Geometry check sheet. Reference: the model listing, model coordinates, mm. Coordinates: 2 decimals unless noted, no trailing zeros. Loops run counter-clockwise (first coordinate to the right, second up) from the corner with the lowest first, then second, coordinate; pieces in that order, holes last.
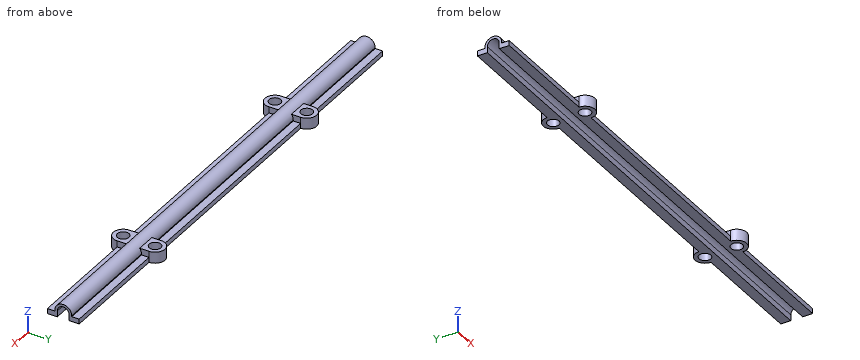
Autodesk Fusion 360 part; units mm, degrees
sketch "Sketch1" plane through (0, 0, 0) normal (1, 0, 0) x (0, 1, 0) in component "CAN_Cable_Cover"
  circle A0 centre (0, 2.4) radius 2.4
  line L0 (-2.4, 2.4) -> (-2.4, 0)
  line L1 (0, 2.5) -> (0, 20)
  line L2 (2.4, 2.4) -> (2.4, 0)
  circle A1 centre (0, 2.4) radius 3.4
  line L3 (-3.4, 2.4) -> (-3.4, 0)
  line L4 (-3.4, 0) -> (-2.4, 0)
  line L5 (3.4, 2.4) -> (3.4, 0)
  line L6 (3.4, 0) -> (2.4, 0)
  line L7 (-3.4, 0) -> (-6.4, 0)
  line L8 (-6.4, 0) -> (-6.4, 2)
  line L9 (-6.4, 2) -> (-3.4, 2)
  line L10 (-3.4, 2) -> (-3.4, 0)
  line L11 (6.4, 2) -> (3.4, 2)
  line L12 (6.4, 0) -> (6.4, 2)
  line L13 (3.4, 0) -> (6.4, 0)
  line L14 (3.4, 2) -> (3.4, 0)
  dimension "d1" = 4.8
  dimension "d2" = 1
  dimension "d5" = 3
  dimension "d6" = 2
extrude "Extrude1" add sketch "Sketch1" along normal mid plane 200 contours A0 L0 L1 A1 L4 | A0 L1 L2 A1 L6 | A1 L3 L4 L10 | A1 L5 L6 L14 | L3 L7 L8 L9 L10 | L5 L11 L12 L13 L14 in component "CAN_Cable_Cover"
sketch "Sketch2" plane through (0, 0, 0) normal (0, 0, -1) x (1, 0, 0) in component "CAN_Cable_Cover"
  line L0 (-100, 2.4) -> (100, 2.4)
  line L1 (100, 2.4) -> (100, 6.4)
  line L2 (100, 6.4) -> (-100, 6.4)
  line L3 (-100, 6.4) -> (-100, 2.4)
  circle A0 centre (-50, 6.4) radius 4
  line L4 (0, -1.75) -> (0, -22.5)
  circle A1 centre (-50, 6.4) radius 2.35
  line L5 (-46, 6.4) -> (-46, 2.4)
  line L6 (-46, 2.4) -> (-50, 2.4)
  line L7 (-54, 6.4) -> (-54, 2.4)
  line L8 (-54, 2.4) -> (-50, 2.4)
  line L9 (1.75, 0) -> (22.5, 0)
  circle A2 centre (-50, -6.4) radius 4
  circle A3 centre (-50, -6.4) radius 2.35
  line L10 (-54, -6.4) -> (-54, -2.4)
  line L11 (-54, -2.4) -> (-50, -2.4)
  line L12 (-46, -2.4) -> (-50, -2.4)
  line L13 (-46, -6.4) -> (-46, -2.4)
  line L14 (46, -2.4) -> (50, -2.4)
  line L15 (54, 6.4) -> (54, 2.4)
  line L16 (54, 2.4) -> (50, 2.4)
  line L17 (46, 6.4) -> (46, 2.4)
  circle A4 centre (50, 6.4) radius 4
  circle A5 centre (50, -6.4) radius 4
  line L18 (54, -6.4) -> (54, -2.4)
  circle A6 centre (50, -6.4) radius 2.35
  line L19 (46, -6.4) -> (46, -2.4)
  circle A7 centre (50, 6.4) radius 2.35
  line L20 (54, -2.4) -> (50, -2.4)
  line L21 (46, 2.4) -> (50, 2.4)
  dimension "d7" = 8
  dimension "d8" = 50
  dimension "d9" = 4.7
extrude "Extrude2" add sketch "Sketch2" against normal blind 4.5 contours L0 A0 L7 L8 | L0 A0 L5 L6 | L2 A0 A1 | L2 A0 A1 | L0 L17 A4 L21 | L2 A4 A7 | L2 A4 A7 | L0 L15 L16 A4 | A2 | A2 L12 L13 | A2 L10 L11 | L14 A5 L19 | A5 L18 L20 | A5 in component "CAN_Cable_Cover"
extrude "Extrude3" cut sketch "Sketch2" against normal blind 16 contours L2 A1 | L2 A7 | A3 | A6 picked at (-50.2862, 5.6708) picked at (49.2594, 5.8292) in component "CAN_Cable_Cover"
component "CAN_Cable_Cover" placed x (1, 0, 0) y (0, 1, 0) z (0, 0, 1) at (0, 0, 0)
equation "d1 = cable_dia"
equation "d2 = tube_thick"
equation "d3 = length"
equation "d4 = 0deg 0'"
equation "d11 = 0deg 0'"
equation "d13 = 0deg 0'"
equation "length = 200 mm"
equation "cable_dia = 4.8 mm"
equation "tube_thick = 1 mm"
1) Depth check by flat-ended pin: pin 1 (6 mm diameter, centred on x = -50, y = -6.4, fed in from +Z); pin 2 (1.2 mm diameter, centred on x = 11, z = 1, fed in from -Y); pin 3 (1.9 mm diameter, centred on x = 41, z = 1.5, fed in from +Y). Enter the tip coordinate at first touch or a pass-through.
Data:
pin 1: stops at z = 4.5
pin 2: stops at y = -6.4
pin 3: stops at y = 6.4
2) Material ranges on probe 1 along Y at (x, z) = (50, 1.55); probe 2 along X at (y, z) = (6.4, 2.8); probe 3 along X at (y, z) = (3, 4.4), recorded low to high.
Data:
probe 1: y = -10.4 to -8.75, -4.05 to -2.4, 2.4 to 4.05, 8.75 to 10.4
probe 2: x = -54 to -52.35, -47.65 to -46, 46 to 47.65, 52.35 to 54
probe 3: x = -54 to -46, 46 to 54
3) Section check B-B on y = 0. Record the cut outline in (x, z).
Data:
outline: (-100, 4.8) - (100, 4.8) - (100, 5.8) - (-100, 5.8) - close
4) Section check A-A on x = 50. Record the cut outline in (y, z), and give its area (3 significant figures).
Data:
outline: (-10.4, 0) - (-8.75, 0) - (-8.75, 4.5) - (-10.4, 4.5) - close; (-4.05, 0) - (-2.4, 0) - (-2.4, 2.4) arc R2.4 cw to (2.4, 2.4) - (2.4, 0) - (4.05, 0) - (4.05, 4.5) - (2.67, 4.5) arc R3.4 ccw to (-2.67, 4.5) - (-4.05, 4.5) - close; (8.75, 0) - (10.4, 0) - (10.4, 4.5) - (8.75, 4.5) - close
area: 35.6 mm2
